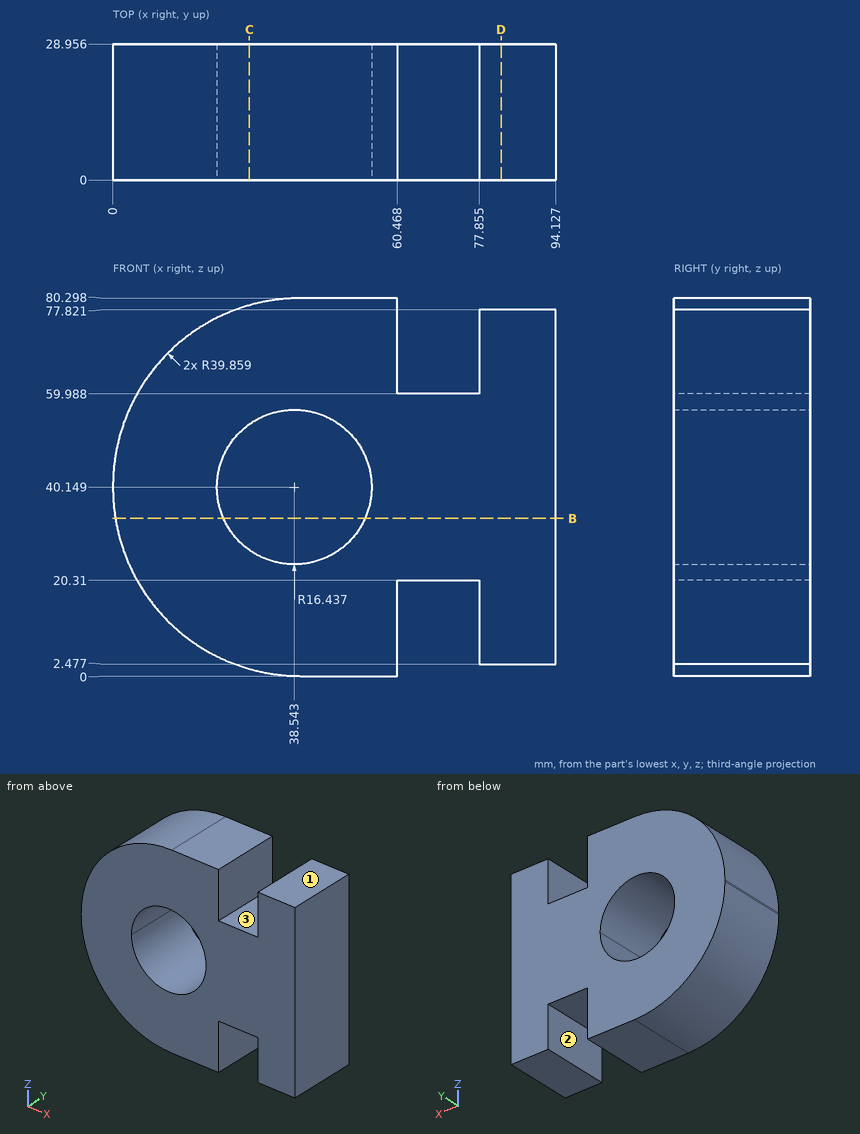
Part print with two shaded views. Sizes in mm from the minimum x, y, z corner. A direction names the side the tool comes from. Round coordinates to 2 decimals unless told otherwise and drop trailing zeros. Write each loop counter-clockwise with the first axis right and the second up, starting at its lowest first coordinate (ties: lowest second). Pieces come first, ordered by that corner, then holes. Notation, with made-up numbers: (34.25, 16) -> (39.25, 16) arc R19 ccw to (39.25, 51) -> close; hole circle Ø7 at (46.25, 30). An arc over 180 degrees is marked (long way). Put each result on its own line as item: value.
Item 1: Slice it at D-D, the plane x = 82.5. Give the cut face in (y, z).
Here are the results:
outline: (0, 2.48) -> (28.96, 2.48) -> (28.96, 77.82) -> (0, 77.82) -> close
Item 2: Slice it at C-C, the plane x = 29. Give the cut face in (y, z), plus the area to 3 significant figures.
Here are the results:
outline: (0, 1.51) -> (28.96, 1.51) -> (28.96, 26.77) -> (0, 26.77) -> close; (0, 53.53) -> (28.96, 53.53) -> (28.96, 78.79) -> (0, 78.79) -> close
area: 1,460 mm^2
Item 3: Tool access for the marked faces 1, 2 and 3: list every direction of +Z, -Z, +X, -X, +Y, -Y with a clear straight run to the whole face (end or side of a thin tool).
Here are the results:
face 1: +Z, +X, +Y, -Y
face 2: -Z, +Y, -Y
face 3: +Z, +Y, -Y
Item 4: Flat gauge pins, fed straight in: P1, Ø5.5, axis at y = 20.5, z = 8, coming from the -X side; P2, Ø9, axis at y = 21, z = 69.5, coming from the -X side (1 decimal); P3, Ø13, axis at x = 88.5, y = 18.5, coming from the +Z side. Where does each tip first touch, or does it go through?
Here are the results:
P1: stops at x = 12.63
P2: stops at x = 8.5
P3: stops at z = 77.82
Item 5: Wall check: probe 1 along Z at (x, y) = (88, 19.5); probe 2 along X at (y, z) = (23.75, 12.5) (1 decimal); probe 3 along X at (y, z) = (3, 10.5) (1 decimal). Give the ranges that are in metal, low to high. Write a range as from..to.
Here are the results:
probe 1: z = 2.48..77.82
probe 2: x = 10.9..60.5, 77.9..94.1
probe 3: x = 12.9..60.5, 77.9..94.1
Item 6: Slice it at B-B, the plane z = 33.5. Give the cut face in (x, y) (1 decimal), plus the area to 3 significant figures.
Here are the results:
outline: (0.5, 0) -> (23.5, 0) -> (23.5, 29) -> (0.5, 29) -> close; (53.6, 0) -> (94.1, 0) -> (94.1, 29) -> (53.6, 29) -> close
area: 1,840 mm^2
